Autodesk Inventor part; units mm, degrees
ref_plane "Work Plane2" through (67.878, 24.3157, 444.5) normal (0, 0, -1) x (-1, 0, 0)
ref_plane "YZ Plane" through (0, 0, 0) normal (1, 0, 0) x (0, 1, 0)
ref_plane "XZ Plane" through (0, 0, 0) normal (0, 1, 0) x (-1, 0, 0)
sketch "Sketch1" plane through (0, 0, 0) normal (0, 0, 1) x (1, 0, 0)
  line L0 (-25.9259, -4.2593) -> (-25.9259, 24.3157)
  line L1 (-25.9259, 24.3157) -> (5.8241, 24.3157)
  line L2 (5.8241, 24.3157) -> (5.8241, -4.2593)
  line L3 (5.8241, -4.2593) -> (2.6491, -4.2593)
  line L4 (2.6491, -4.2593) -> (2.6491, 21.1407)
  line L5 (2.6491, 21.1407) -> (-22.7509, 21.1407)
  line L6 (-22.7509, 21.1407) -> (-22.7509, -4.2593)
  line L7 (-22.7509, -4.2593) -> (-25.9259, -4.2593)
  dimension "d0" = 25.4
  dimension "d1" = 31.75
  dimension "d2" = 3.175
  dimension "d3" = 3.175
  dimension "d4" = 28.575
  dimension "d5" = 0
extrude "Extrusion1" add sketch "Sketch1" along normal blind 889
fillet "Fillet1" radius 6.35 4 edges at (-22.7509, 21.1407, 444.5) (-25.9259, 24.3157, 444.5) (5.8241, 24.3157, 444.5) (2.6491, 21.1407, 444.5)
fillet "Fillet2" radius 3.175 4 edges at (4.2366, -4.2593, 889) (-24.3384, -4.2593, 889) (-24.3384, -4.2593, 0) (4.2366, -4.2593, 0)
sketch "Sketch2" plane through (-25.9259, 17.9657, 0) normal (-1, 0, 0) x (0, 0, 1)
  line L0 (3.175, -22.225) -> (885.825, -22.225)
  line L1 (0, -19.05) -> (0, 0)
  circle A0 centre (12.7, -9.525) radius 3.175
  dimension "d10" = 6.35
  dimension "d11" = 12.7
  dimension "d12" = 12.7
extrude "Extrusion2" cut sketch "Sketch2" against normal through all
pattern_linear "Rectangular Pattern1" count 35 spacing 25.4 along (0, 0, 1) of "Extrusion2"
ref_plane "Work Plane2" through (67.878, 24.3157, 444.5) normal (0, 0, -1) x (-1, 0, 0)
sketch "Sketch6" plane through (5.8241, 17.9657, 889) normal (1, 0, 0) x (0, 0, -1)
  circle A0 centre (698.5, -9.525) radius 3.175
  circle A1 centre (723.9, -9.525) radius 3.175
  circle A2 centre (749.3, -9.525) radius 3.175
  circle A3 centre (774.7, -9.525) radius 3.175
  circle A4 centre (800.1, -9.525) radius 3.175
  circle A5 centre (825.5, -9.525) radius 3.175
  circle A6 centre (850.9, -9.525) radius 3.175
  circle A7 centre (876.3, -9.525) radius 3.175
  line L0 (976.9561, 155.027) -> (631.825, 155.027)
  line L1 (631.825, 155.027) -> (631.825, -109.3216)
  line L2 (631.825, -109.3216) -> (976.9561, -109.3216)
  line L3 (976.9561, -109.3216) -> (976.9561, 155.027)
  line L4 (0, 0) -> (0, -19.05)
  dimension "d54" = 631.825
extrude "Extrusion5" cut sketch "Sketch6" against normal through all
sketch "Sketch8" plane through (-19.5759, 24.3157, 889) normal (0, 1, 0) x (1, 0, 0)
  line L0 (19.05, 631.825) -> (0, 631.825)
  line L1 (0, 0) -> (19.05, 0)
  circle A0 centre (9.525, 82.55) radius 3.175
  circle A1 centre (9.525, 107.95) radius 3.175
  circle A2 centre (9.525, 184.15) radius 3.175
  circle A3 centre (9.525, 234.95) radius 3.175
  circle A4 centre (9.525, 549.275) radius 3.175
  circle A5 centre (9.525, 396.875) radius 3.175
  circle A6 centre (9.525, 523.875) radius 3.175
  circle A7 centre (9.525, 447.675) radius 3.175
  point P0 (19.5759, 889)
  point P1 (9.525, 0)
  dimension "d43" = 6.35
  dimension "d44" = 82.55
  dimension "d45" = 25.4
  dimension "d46" = 76.2
  dimension "d47" = 50.8
  dimension "d48" = 82.55
  dimension "d49" = 25.4
  dimension "d50" = 76.2
  dimension "d51" = 50.8
extrude "Extrusion7" cut sketch "Sketch8" along normal through all both and the other way through all
sketch "Sketch9" plane through (5.8241, -4.2593, 257.175) normal (0, -1, 0) x (1, 0, 0)
  line L0 (-3.175, 0) -> (0, 0)
  line L1 (0, 0) -> (0, 628.65)
  line L2 (-3.175, 628.65) -> (0, 628.65)
  line L3 (-3.175, 0) -> (-3.175, 628.65)
  line L4 (-31.75, 0) -> (-28.575, 0)
  line L5 (-28.575, 0) -> (-28.575, 628.65)
  line L6 (-31.75, 628.65) -> (-28.575, 628.65)
  line L7 (-31.75, 0) -> (-31.75, 628.65)
  point P0 (-5.8241, -257.175)
sketch "Sketch10" plane through (-25.9259, -1.0843, 889) normal (-1, 0, 0) x (0, 0, 1)
  circle A0 centre (-304.8, 9.525) radius 3.175
  circle A1 centre (-330.2, 9.525) radius 3.175
  circle A2 centre (-304.8, 9.525) radius 3.175
  circle A3 centre (-330.2, 9.525) radius 3.175
  circle A4 centre (-279.4, 9.525) radius 3.175
  circle A5 centre (-355.6, 9.525) radius 3.175
  point P0 (-889, 1.0843)
  dimension "d55" = 6.35
  dimension "d56" = 6.35
  dimension "d57" = 25.4
  dimension "d58" = 50.8
extrude "Extrusion8" cut sketch "Sketch10" against normal blind 38.1
sketch "Sketch11" plane through (0, 0, 889) normal (0, 0, 1) x (1, 0, 0)
  line L0 (-22.7509, -1.0843) -> (-25.9259, -1.0843)
  line L1 (-22.7509, 14.7907) -> (-22.7509, -1.0843)
  arc A0 (-16.4009, 21.1407) -> (-22.7509, 14.7907) centre (-16.4009, 14.7907) ccw
  line L2 (-3.7009, 21.1407) -> (-16.4009, 21.1407)
  arc A1 (2.6491, 14.7907) -> (-3.7009, 21.1407) centre (-3.7009, 14.7907) ccw
  line L3 (2.6491, -1.0843) -> (2.6491, 14.7907)
  line L4 (5.8241, -1.0843) -> (2.6491, -1.0843)
  line L5 (5.8241, 17.9657) -> (5.8241, -1.0843)
  arc A2 (5.8241, 17.9657) -> (-0.5259, 24.3157) centre (-0.5259, 17.9657) ccw
  line L6 (-19.5759, 24.3157) -> (-0.5259, 24.3157)
  arc A3 (-19.5759, 24.3157) -> (-25.9259, 17.9657) centre (-19.5759, 17.9657) ccw
  line L7 (-25.9259, -1.0843) -> (-25.9259, 17.9657)
  line L8 (-25.9259, -4.2593) -> (-22.7509, -4.2593)
  line L9 (2.6491, -4.2593) -> (5.8241, -4.2593)
  line L10 (-90.542, -90.1503) -> (-1.8937, -1.502)
  line L11 (-25.9259, 17.9657) -> (-25.9259, -25.5343)
  line L12 (4.9313, -8.327) -> (-83.0857, -96.3441)
  line L13 (-25.9259, 17.9657) -> (-25.9259, -39.1843)
  line L14 (-19.5759, 24.3157) -> (-31.8681, 24.3157)
  line L15 (-25.9259, 24.3157) -> (-25.9259, -39.1843)
  point P0 (0, 0)
  dimension "d61" = 49.85
  dimension "d62" = 63.5
properties part number "C Channel 2 1764"
Work out the finished part from the listing and answer in its coordinate system (mm). A direction names the side the tool comes from. Give positions to 0.01 mm unless a question says otherwise; leave off trailing zeros. Order: outer loops, then holes, each group sorted by start corner. A loop starts at its lowest first (then second) coordinate and runs counter-clockwise, first axis right, second up. Notation, with made-up numbers: (16.25, 55.25) -> (60.25, 55.25) arc R24 cw to (60.25, 74.25) -> close; hole circle Ø8 at (83, 21). An arc over 180 degrees is marked (long way). Answer as a JSON object with one key per item and string values. Group by question number.
1. Flat-ended cylindrical pins translate along their axes: pin 1 Ø10 at (y, z) = (8.44, 647.7) entering from +X; pin 2 Ø5 at (y, z) = (8.44, 850.9) entering from -X; pin 3 Ø3 at (x, z) = (-7, 530.5) entering from -Y; pin 4 Ø5 at (x, z) = (-17, 518) entering from -Y. Find the tip coordinate at first contact, or state that the pin passes through.
2. Section A-A on z = 732.5 is taken. Determine the outline of the cut face in (x, y).
3. A tool of negligible diameter and unlimited length cuts with its end or side. For faces 1 (the flat face through (-10, 21.141, 569)), 2 (the flat face through (-10, 22, 889)), from which of +Z, -Z, +X, -X, +Y, -Y can it reach the whole face along a straight path? Write none if from no direction.
4. Consider line 1 along X through (y, z) = (1, 854); line 2 along Y through (x, z) = (-17, 666.5); line 3 along X through (y, z) = (15.25, 469.5). Determine where each line is inside the solid, lowest interval first. Write a range as [from, to].
5. The mould has two halves that part along X. Classify faces 3 (the flat face through (-22.751, 5, 569)), 4 (the flat face through (-10, 24.316, 569)), 5 (the flat face through (5.824, 5, 569)), 6 (the flat face through (2.649, 5, 569)): released by +X, released by -X, zero draft, split by the parting line, or undercut.
Result sheet:
{
 "1": {"pin 1": "stops at x = 5.82", "pin 2": "passes through", "pin 3": "stops at y = 21.14", "pin 4": "stops at y = 20.33"},
 "2": {"outline": "(-25.93, -4.26) -> (-22.75, -4.26) -> (-22.75, 14.79) arc R6.35 cw to (-16.4, 21.14) -> (-3.7, 21.14) arc R6.35 cw to (2.65, 14.79) -> (2.65, -4.26) -> (5.82, -4.26) -> (5.82, 17.97) arc R6.35 ccw to (-0.53, 24.32) -> (-19.58, 24.32) arc R6.35 ccw to (-25.93, 17.97) -> close"},
 "3": {"face 1": "+Z, -Z, -Y", "face 2": "+Z, +X, -X, +Y, -Y"},
 "4": {"line 1": "x = [-25.93, -22.75], [2.65, 5.82]", "line 2": "y = [21.11, 24.32]", "line 3": "x = [-25.93, -22.73], [2.63, 5.82]"},
 "5": {"face 3": "undercut", "face 4": "zero draft", "face 5": "released by +X", "face 6": "undercut"}
}
